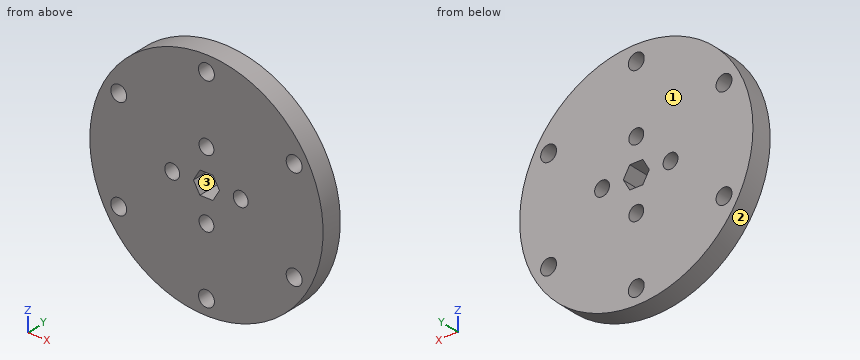
Autodesk Inventor part; units mm, degrees
ref_plane "Work Plane5" through (0, 21.082, 0) normal (0, 1, 0) x (1, 0, 0)
ref_plane "Work Plane6" through (0, 21.082, 0) normal (0, 1, 0) x (1, 0, 0)
ref_plane "YZ Plane" through (0, 0, 0) normal (1, 0, 0) x (0, 1, 0)
sketch "Sketch1" plane through (0, 0, 0) normal (0, 1, 0) x (-1, 0, 0)
  circle A0 centre (0, 0) radius 27.94
  dimension "d0" = 55.88
extrude "Extrusion1" add sketch "Sketch1" along normal blind 7.62
ref_plane "Work Plane5" through (0, 21.082, 0) normal (0, 1, 0) x (1, 0, 0)
sketch "Sketch5" plane through (0, 21.082, 0) normal (0, 1, 0) x (1, 0, 0)
  line L0 (0, 0) -> (0, 2.667)
  line L1 (-3.1168, 0) -> (-1.5584, 2.6992)
  line L2 (-1.5584, 2.6992) -> (1.5584, 2.6992)
  line L3 (1.5584, 2.6992) -> (3.1168, 0)
  line L4 (3.1168, 0) -> (1.5584, -2.6992)
  line L5 (1.5584, -2.6992) -> (-1.5584, -2.6992)
  line L6 (-1.5584, -2.6992) -> (-3.1168, 0)
  dimension "d10" = 2.667
extrude "Extrusion4" cut sketch "Sketch5" against normal blind 25.4
sketch "Sketch6" plane through (0, 7.62, 0) normal (0, 1, 0) x (1, 0, 0)
  circle A0 centre (0, 0) radius 27.94
  line L0 (0, -27.94) -> (0, -26.162)
  line L1 (0, -26.162) -> (0, -24.257)
  circle A1 centre (0, -24.257) radius 1.905
  dimension "d13" = 1.778
  dimension "d14" = 1.905
extrude "Extrusion5" cut sketch "Sketch6" against normal blind 25.4 contours A1
ref_plane "Work Plane6" through (0, 21.082, 0) normal (0, 1, 0) x (1, 0, 0)
pattern_circular "Circular Pattern1" count 6 over 360 about axis through (0, 21.082, 0) along (0, 1, 0) of "Extrusion5"
sketch "Sketch8" plane through (0, 0, 0) normal (0, -1, 0) x (1, 0, 0)
  line L0 (3.1168, 0) -> (1.5584, -2.6992)
  line L1 (3.1168, 0) -> (6.4188, 0)
  line L2 (6.4188, 0) -> (8.1968, 0)
  circle A0 centre (8.1968, 0) radius 1.778
  point P0 (0, 0)
  dimension "d20" = 3.302
  dimension "d21" = 1.778
extrude "Extrusion6" cut sketch "Sketch8" against normal blind 25.4
pattern_circular "Circular Pattern2" count 4 over 360 about axis through (0, 21.082, 0) along (0, 1, 0) of "Extrusion6"
sketch "Sketch10" plane through (0, 7.62, 0) normal (0, 1, 0) x (1, 0, 0)
  circle A0 centre (0, 0) radius 27.94
extrude "Extrusion8" cut sketch "Sketch10" against normal blind 2.54
properties part number "Wheel Mount"
Can you work these out from the model? Positions are in its coordinate system, mm. Face numbers are marked on the shaded views. Give positions to 0.01 mm unless a question says otherwise; leave off trailing zeros. Order: outer loops, then holes, each group sorted by start corner. A loop starts at its lowest first (then second) coordinate and runs counter-clockwise, first axis right, second up. Notation, with made-up numbers: M 61.5,85 L 75.5,85 A8 ccw 75.5,93 Z; hole C 8.5,59 d4. An arc over 180 degrees is marked long. One line per question, with ' | ' between items.
Item 1: Please list where these lines run through material, in increasing order: L1, parallel to X at y = 1.15, z = 0; L2, parallel to Z at x = 21, y = 3.25; L3, parallel to Z at x = 20, y = 4.5.
Answer block:
L1: x = -27.94 to -9.97, -6.42 to -3.12, 3.12 to 6.42, 9.97 to 27.94 | L2: z = -18.43 to -14.03, -10.22 to 10.22, 14.03 to 18.43 | L3: z = -19.51 to -13.75, -10.51 to 10.51, 13.75 to 19.51
Item 2: Suppose I cut it at A-A, the plane x = 0. Write out the boundary of the cut face in (y, z), then the cut area to 3 significant figures.
Answer block:
outline: M 0,-27.94 L 5.08,-27.94 L 5.08,-26.16 L 0,-26.16 Z; M 0,-22.35 L 5.08,-22.35 L 5.08,-9.97 L 0,-9.97 Z; M 0,-6.42 L 5.08,-6.42 L 5.08,-2.7 L 0,-2.7 Z; M 0,2.7 L 5.08,2.7 L 5.08,6.42 L 0,6.42 Z; M 0,9.97 L 5.08,9.97 L 5.08,22.35 L 0,22.35 Z; M 0,26.16 L 5.08,26.16 L 5.08,27.94 L 0,27.94 Z | area: 182 mm2
Item 3: Suppose I cut it at B-B, the plane x = -21. Write out the boundary of the cut face in (y, z), then the cut area to 3 significant figures.
Answer block:
outline: M 0,-18.43 L 5.08,-18.43 L 5.08,-14.03 L 0,-14.03 Z; M 0,-10.22 L 5.08,-10.22 L 5.08,10.22 L 0,10.22 Z; M 0,14.03 L 5.08,14.03 L 5.08,18.43 L 0,18.43 Z | area: 149 mm2
Item 4: We'd pull the mould along X, two halves only. Please class the marked faces 1, 2 and 3: released by +X, released by -X, zero draft, split by the parting line, or undercut.
Answer block:
face 1: zero draft | face 2: split by the parting line | face 3: undercut
Item 5: I'm going to push flat-ended pins straight in: pin 1 Ø4.5 at (x, z) = (0, -24.257) entering from -Y; pin 2 Ø3.5 at (x, z) = (0, 24.257) entering from +Y; pin 3 Ø0.9 at (x, y) = (0, 3.5) entering from +Z. Where does each tip first touch, or does it pass through?
Answer block:
pin 1: stops at y = 0 | pin 2: passes through | pin 3: stops at z = 27.94
Item 6: Suppose I cut it at D-D, the plane y = 3.95. Give the number of separate pieces and of enclosed holes in the cut face, then the cut area to 3 significant figures.
Answer block:
separate pieces: 1 | enclosed holes: 11 | area: 2,320 mm2
Item 7: Suppose I cut it at C-C, the plane z = 1. Write out the boundary of the cut face in (x, y), then the cut area to 3 significant figures.
Answer block:
outline: M -27.92,0 L -9.67,0 L -9.67,5.08 L -27.92,5.08 Z; M -6.73,0 L -2.54,0 L -2.54,5.08 L -6.73,5.08 Z; M 2.54,0 L 6.73,0 L 6.73,5.08 L 2.54,5.08 Z; M 9.67,0 L 27.92,0 L 27.92,5.08 L 9.67,5.08 Z | area: 228 mm2
